For this review, use the dimensioned drawing (mm, ordinates from the lowest corner) and the shaded views. A direction names the side the tool comes from. Round coordinates to 2 decimals unless told otherwise and drop trailing zeros. Write each loop counter-clockwise with the first axis right and the second up, starting at its lowest first coordinate (ties: lowest second). Pieces come first, ordered by that corner, then holes. Notation, with made-up numbers: M -30.75,14 L -10.75,14 A34 ccw -10.75,50 Z; hole C 35.25,-34 d4. An arc over 180 degrees is marked long. One line per question, with ' | ' between items. Start each with the question number.
Item 1: Add section B-B, the plane z = 74.5. State the section outline as (x, y) points, and give its area (3 significant figures).
Item 2: Insertion check: pin 1 Ø4 at (x, y) = (31, 28) entering from -Z; pin 2 Ø23 at (y, z) = (36.5, 47) entering from +X; pin 3 Ø12.5 at (y, z) = (52, 17) entering from +X; pin 4 Ø7.5 at (x, z) = (24, 95) entering from -Y. Each pin has a flat end and moves straight along its axis. Give the tip position at first contact, or say it passes through.
Item 3: Add section A-A, the plane x = 116.5. State the section outline as (y, z) points, and give its area (3 significant figures).
Item 4: Machinability: for the marked faces 1, 2 and 3, which of the approach directions +Z, -Z, +X, -X, +Y, -Y give a long, thin tool a straight path to every point of the face, cutting with its end or side? Answer none if there is none.
Item 5: For L1, parallel to X at y = 80.5, z = 43.5; L2, parallel to Z at x = 67, y = 61; L3, parallel to X at y = 33.5, z = 17, list the stretches that pass through material, from the lowest coordinate up.
Item 6: Draft analysis for pull direction Y (two halves, no side actions). For the marked faces 4, 5 and 6, state which applies: released by +Y, released by -Y, zero draft, split by the parting line, or undercut.
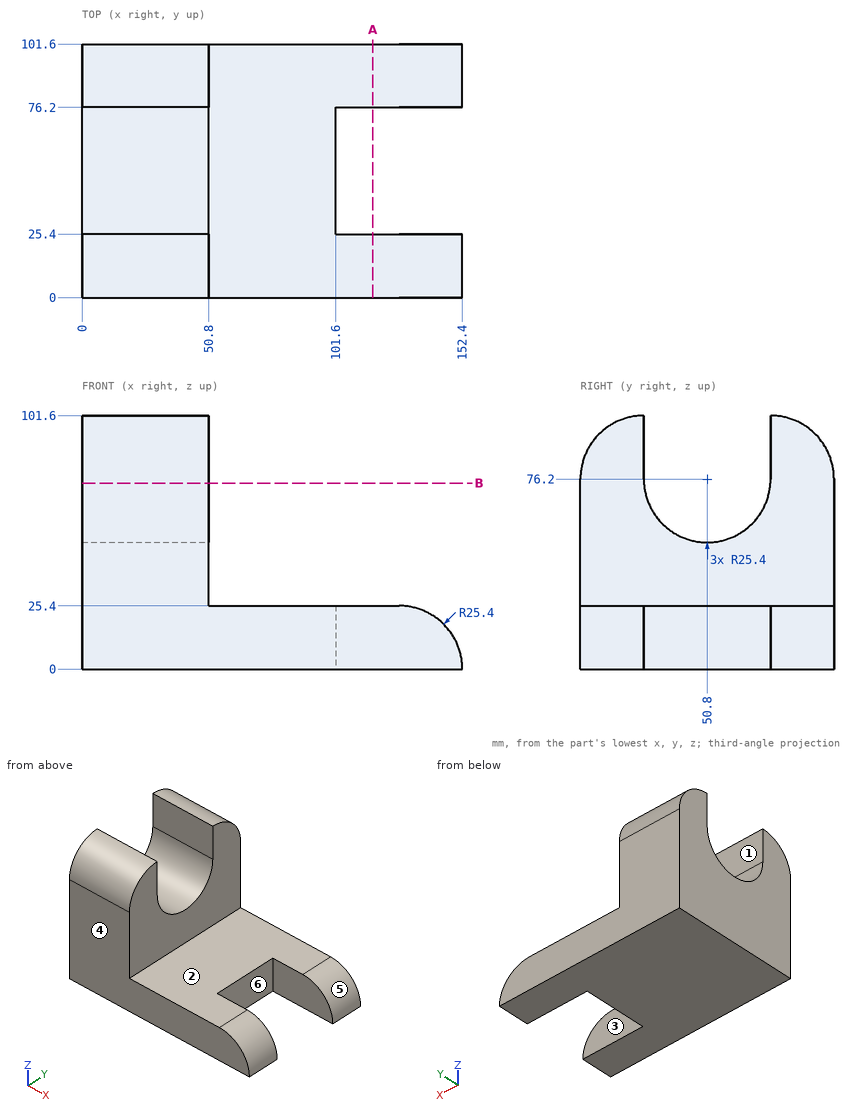
Computed values:
1) outline: M 0,0 L 50.8,0 L 50.8,25.46 L 0,25.46 Z; M 0,76.14 L 50.8,76.14 L 50.8,101.6 L 0,101.6 Z | area: 2,590 mm^2
2) pin 1: stops at z = 0 | pin 2: stops at x = 50.8 | pin 3: stops at x = 101.6 | pin 4: stops at y = 4.94
3) outline: M 0,0 L 25.4,0 L 25.4,25.4 L 0,25.4 Z; M 76.2,0 L 101.6,0 L 101.6,25.4 L 76.2,25.4 Z | area: 1,290 mm^2
4) face 1: +Z, +X, -X | face 2: +Z, +X, +Y, -Y | face 3: +Z, -Z, +X
5) L1: x = 0 to 50.8 | L2: z = 0 to 25.4 | L3: x = 0 to 101.6
6) face 4: released by -Y | face 5: zero draft | face 6: undercut
